Design review of the part built by this model. Coordinates are the model's own, in mm. Give positions to 0.01 mm unless a question says otherwise; leave off trailing zeros. Loops run counter-clockwise (first coordinate to the right, second up) from the corner with the lowest first, then second, coordinate; pieces in that order, holes last. Notation, with made-up numbers: M 3.25,52.25 L 48.25,52.25 A22 ccw 48.25,72.25 Z; hole C 44.25,72.25 d9. An arc over 180 degrees is marked long. Answer as CSV lines item,"result".
```python
from build123d import *

# Parameters (mm, degrees)
SKETCH1_W           = 70
SKETCH1_H           = 13.5
BOSS_EXTRUDE1_DEPTH = 50
SKETCH2_W           = 34
SKETCH2_H           = 10
CUT_EXTRUDE1_DEPTH  = 100
SKETCH3_R           = 3.225
CUT_EXTRUDE2_DEPTH  = 3
CHAMFER1_SIZE       = 0.5
SKETCH4_R           = 4.15
CUT_EXTRUDE3_DEPTH  = 5
SKETCH5_R           = 3.15
CUT_EXTRUDE4_DEPTH  = 3
CHAMFER2_SIZE       = 3
CHAMFER3_SIZE       = 5


with BuildPart() as part:
    # Sketch1 → Boss-Extrude1 (new, symmetric)
    with BuildSketch(Plane(origin=(0, 0, 0), x_dir=(1, 0, 0), z_dir=(0, 1, 0))):
        Rectangle(SKETCH1_W, SKETCH1_H)
    extrude(amount=BOSS_EXTRUDE1_DEPTH, both=True)

    # Sketch2 → Cut-Extrude1 (cut)
    with BuildSketch(Plane.XY.offset(6.75)):
        with Locations((0, -45)):
            Rectangle(SKETCH2_W, SKETCH2_H)
    extrude(amount=-CUT_EXTRUDE1_DEPTH, mode=Mode.SUBTRACT)

    # Sketch3 → Cut-Extrude2 (cut)
    with BuildSketch(Plane.XZ.offset(40)):
        with Locations(Location((-10, 0, 0), (0, 0, 270))):
            Circle(SKETCH3_R)
        with Locations(Location((0, 0, 0), (0, 0, 270))):
            Circle(SKETCH3_R)
        with Locations(Location((10, 0, 0), (0, 0, 270))):
            Circle(SKETCH3_R)
    extrude(amount=-CUT_EXTRUDE2_DEPTH, mode=Mode.SUBTRACT)

    # Chamfer1
    chamfer1_edges = [part.edges().sort_by_distance(p)[0] for p in [
        (-10, -40, 3.225),
        (0, -40, 3.225),
        (10, -40, 3.225),
    ]]
    chamfer(chamfer1_edges, length=CHAMFER1_SIZE)

    # Sketch4 → Cut-Extrude3 (cut)
    with BuildSketch(Plane.XY.offset(6.75)):
        with Locations((-23.33, 42)):
            Circle(SKETCH4_R)
        with Locations((-11.66, 42)):
            Circle(SKETCH4_R)
        with Locations((0.01, 42)):
            Circle(SKETCH4_R)
        with Locations((11.68, 42)):
            Circle(SKETCH4_R)
        with Locations((23.35, 42)):
            Circle(SKETCH4_R)
    extrude(amount=-CUT_EXTRUDE3_DEPTH, mode=Mode.SUBTRACT)

    # Sketch5 → Cut-Extrude4 (cut)
    with BuildSketch(Plane.XY.offset(1.75)):
        with Locations((-23.33, 42)):
            Circle(SKETCH5_R)
        with Locations((-11.66, 42)):
            Circle(SKETCH5_R)
        with Locations((0.01, 42)):
            Circle(SKETCH5_R)
        with Locations((11.68, 42)):
            Circle(SKETCH5_R)
        with Locations((23.35, 42)):
            Circle(SKETCH5_R)
    extrude(amount=-CUT_EXTRUDE4_DEPTH, mode=Mode.SUBTRACT)

    # Chamfer2
    chamfer2_edges = [part.edges().sort_by_distance(p)[0] for p in [
        (17, -50, 0),
        (-17, -50, 0),
        (-35, -50, 0),
        (35, -50, 0),
    ]]
    chamfer(chamfer2_edges, length=CHAMFER2_SIZE)

    # Chamfer3
    chamfer3_edges = [part.edges().sort_by_distance(p)[0] for p in [
        (-35, 50, 0),
        (35, 50, 0),
    ]]
    chamfer(chamfer3_edges, length=CHAMFER3_SIZE)


solid = part.part
```
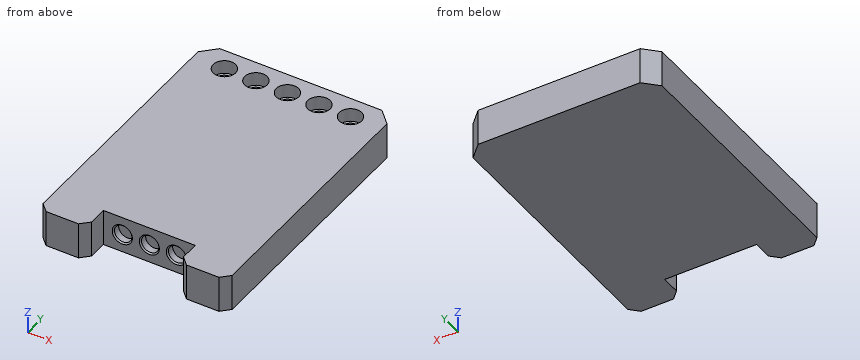
1. We need section C-C, the plane x = 10. Write out the cut boundary in (y, z) (3 decimals), plus the area to 3 significant figures.
Answer block:
outline,"M -40,-6.75 L 50,-6.75 L 50,6.75 L 45.795,6.75 L 45.795,1.75 L 44.665,1.75 L 44.665,-1.25 L 39.335,-1.25 L 39.335,1.75 L 38.205,1.75 L 38.205,6.75 L -40,6.75 L -40,3.725 L -39.5,3.225 L -37,3.225 L -37,-3.225 L -39.5,-3.225 L -40,-3.725 Z"
area,"1,140 mm²"
2. For P1, Ø3, axis at x = -1, y = 41.5, coming from the +Z side; P2, Ø1, axis at x = 13, z = -3.5, coming from the -Y side; P3, Ø5, axis at x = -10, z = 0, coming from the -Y side, all flat-tipped, find the tip position at first contact; note any pin that passes through.
Answer block:
P1,"z = -1.25"
P2,"y = -40"
P3,"y = -37"
3. We need section A-A, the plane z = 5.5. Write out the cut boundary in (x, y), plus the area to 3 significant figures.
Answer block:
outline,"M -35,-47 L -32,-50 L -20,-50 L -17,-47 L -17,-40 L 17,-40 L 17,-47 L 20,-50 L 32,-50 L 35,-47 L 35,45 L 30,50 L -30,50 L -35,45 Z; hole C -23.33,42 d8.3; hole C -11.66,42 d8.3; hole C 0.01,42 d8.3; hole C 11.68,42 d8.3; hole C 23.35,42 d8.3"
area,"6,350 mm²"
4. To check wall thickness, follow L1, parallel to X at y = -38.25, z = 0 (3 decimals); L2, parallel to Y at x = -11.66, z = 0.35; L3, parallel to X at y = -44, z = 5.25. State the ranges of each line that lie inside material, in increasing order. Write a range as [from, to].
Answer block:
L1,"[-35, -13.225], [-6.775, -3.225], [3.225, 6.775], [13.225, 35]"
L2,"[-37, 38.85], [45.15, 50]"
L3,"[-35, -17], [17, 35]"
5. We need section B-B, the plane x = -23.33. Write out the cut boundary in (y, z).
Answer block:
outline,"M -50,-6.75 L 50,-6.75 L 50,6.75 L 46.15,6.75 L 46.15,1.75 L 45.15,1.75 L 45.15,-1.25 L 38.85,-1.25 L 38.85,1.75 L 37.85,1.75 L 37.85,6.75 L -50,6.75 Z"
6. We need section D-D, the plane x = -10. Write out the cut boundary in (y, z) (3 decimals), plus the area to 3 significant figures.
Answer block:
outline,"M -40,-6.75 L 50,-6.75 L 50,6.75 L 45.804,6.75 L 45.804,1.75 L 44.677,1.75 L 44.677,-1.25 L 39.323,-1.25 L 39.323,1.75 L 38.196,1.75 L 38.196,6.75 L -40,6.75 L -40,3.725 L -39.5,3.225 L -37,3.225 L -37,-3.225 L -39.5,-3.225 L -40,-3.725 Z"
area,"1,140 mm²"
